Job drawing, mm, ordinate dimensions from the low corner. One solid piece. Round coordinates to 2 decimals unless told otherwise and drop trailing zeros. Loops run counter-clockwise (first coordinate to the right, second up) from the corner with the lowest first, then second, coordinate; pieces in that order, holes last.
1) Mould opens along Z. For the marked faces 1, 2, 3 and 4 say: +Z half, -Z half, draft (parallel to the pull), parting line (faces both ways), or undercut.
2) Band-saw the part on D-D, the plane x = 28. Write the cut outline in (y, z).
3) Band-saw the part on A-A, the plane x = 20. Write the cut outline in (y, z).
4) Band-saw the part on B-B, the plane y = 13. Write the cut outline in (x, z).
5) Band-saw the part on C-C, the plane z = 1. Write the cut outline in (x, y), then the cut area to 3 significant figures.
6) Drop flat-ended pins along their axis: P1, Ø3, axis at x = 21.5, z = 12, coming from the -Y side; P2, Ø1.5, axis at x = 14, y = 16.5, coming from the +Z side; P3, Ø1.6, axis at x = 14, z = 5, coming from the +Y side; P4, Ø1.3, axis at x = 12.5, y = 1, coming from the -Z side. Give the stop position or say it passes through.
7) Probe line 1 (Z direction, x = 28, y = 20.25); line 2 (X direction, y = 19.75, z = 12); line 3 (Y direction, x = 20, z = 7). List the from-to ranges inside material, lowest first.
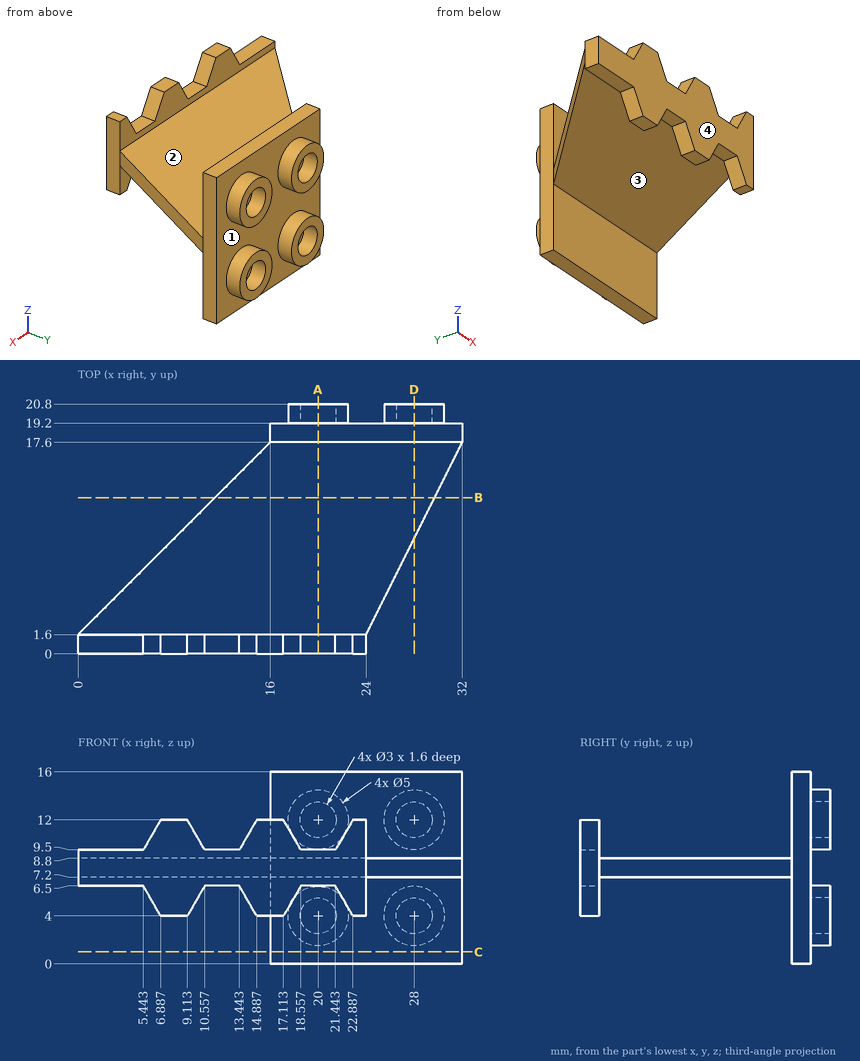
Reported:
1. face 1: undercut
1. face 2: +Z half
1. face 3: -Z half
1. face 4: draft
2. outline: (9.6, 7.2) - (17.6, 7.2) - (17.6, 0) - (19.2, 0) - (19.2, 1.5) - (20.8, 1.5) - (20.8, 2.5) - (19.2, 2.5) - (19.2, 5.5) - (20.8, 5.5) - (20.8, 6.5) - (19.2, 6.5) - (19.2, 9.5) - (20.8, 9.5) - (20.8, 10.5) - (19.2, 10.5) - (19.2, 13.5) - (20.8, 13.5) - (20.8, 14.5) - (19.2, 14.5) - (19.2, 16) - (17.6, 16) - (17.6, 8.8) - (9.6, 8.8) - close
3. outline: (0, 6.5) - (1.6, 6.5) - (1.6, 7.2) - (17.6, 7.2) - (17.6, 0) - (19.2, 0) - (19.2, 1.5) - (20.8, 1.5) - (20.8, 2.5) - (19.2, 2.5) - (19.2, 5.5) - (20.8, 5.5) - (20.8, 6.5) - (19.2, 6.5) - (19.2, 9.5) - (20.8, 9.5) - (20.8, 10.5) - (19.2, 10.5) - (19.2, 13.5) - (20.8, 13.5) - (20.8, 14.5) - (19.2, 14.5) - (19.2, 16) - (17.6, 16) - (17.6, 8.8) - (1.6, 8.8) - (1.6, 9.5) - (0, 9.5) - close
4. outline: (11.4, 7.2) - (29.7, 7.2) - (29.7, 8.8) - (11.4, 8.8) - close
5. outline: (16, 17.6) - (32, 17.6) - (32, 19.2) - (16, 19.2) - close
5. area: 25.6 mm2
6. P1: stops at y = 0
6. P2: stops at z = 8.8
6. P3: stops at y = 1.6
6. P4: stops at z = 6.5
7. line 1: z = 1.5 to 2.5, 5.5 to 6.5, 9.5 to 10.5, 13.5 to 14.5
7. line 2: x = 17.5 to 18.5, 21.5 to 22.5, 25.5 to 26.5, 29.5 to 30.5
7. line 3: y = 0 to 1.6, 17.6 to 19.2
